Read the model definition and answer for the solid it produces. Units are mm, in the model's axes. Face numbers are marked on the shaded views. A direction names the side the tool comes from. Coordinates: 2 decimals unless noted, no trailing zeros. Write each loop counter-clockwise with the first axis right and the second up, starting at its lowest first coordinate (ties: lowest second). Pieces come first, ordered by that corner, then holes. Notation, with made-up numbers: M -9,-22 L 29,-22 A16 cw 29,-6 Z; hole C 23.25,31 d4. An arc over 180 degrees is marked long. Write item = value, one per line.
Autodesk Inventor part; units mm, degrees
ref_plane "YZ Plane" through (0, 0, 0) normal (1, 0, 0) x (0, 1, 0)
ref_plane "XZ Plane" through (0, 0, 0) normal (0, 1, 0) x (-1, 0, 0)
ref_plane "XY Plane" through (0, 0, 0) normal (0, 0, 1) x (1, 0, 0)
sketch "Skizze1" plane through (0, 0, 0) normal (0, 1, 0) x (-1, 0, 0)
  circle A0 centre (36.1244, -29.8236) radius 25
  circle A1 centre (36.1244, -29.8236) radius 1.5
  circle A2 centre (36.1244, -29.8236) radius 20
  point P0 (0, 0)
  dimension "d0" = 50
  dimension "d1" = 40
  dimension "d2" = 3
extrude "Extrusion1" add sketch "Skizze1" along normal blind 5 and the other way blind 5 contours A0
extrude "Extrusion2" add sketch "Skizze1" along normal blind 2.5 and the other way blind 2.5 contours A2
properties part number "Rad"
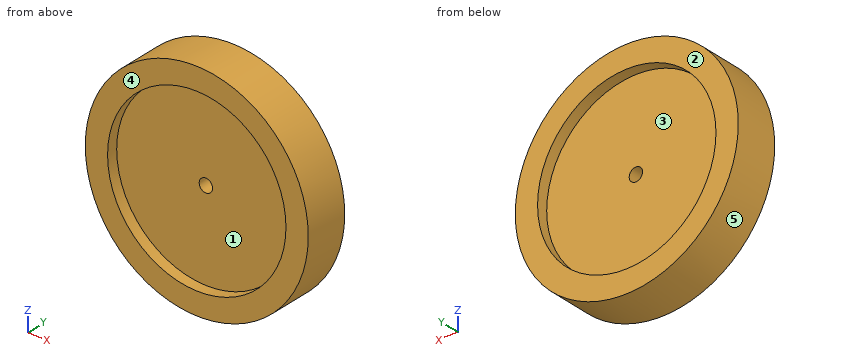
Item 1: Find section B-B (x = -30). Determine the outline of the cut face in (y, z).
Worked answers:
outline = M -5,-54.06 L 5,-54.06 L 5,-48.86 L 2.5,-48.86 L 2.5,-10.78 L 5,-10.78 L 5,-5.59 L -5,-5.59 L -5,-10.78 L -2.5,-10.78 L -2.5,-48.86 L -5,-48.86 Z
Item 2: Find section D-D (y = 1.5). Determine the outline of the cut face in (x, z), and give its area (3 significant figures).
Worked answers:
outline = C -36.12,-29.82 d50; hole C -36.12,-29.82 d3
area = 1,960 mm²
Item 3: Find section C-C (y = 4). Determine the outline of the cut face in (x, z).
Worked answers:
outline = C -36.12,-29.82 d50; hole C -36.12,-29.82 d40
Item 4: For a pull along Z with two mould halves and no side action, classify the marked faces 3, 4 and 5 as released by +Z, released by -Z, zero draft, split by the parting line, or undercut.
Worked answers:
face_3 = undercut
face_4 = zero draft
face_5 = split by the parting line
Item 5: Find section A-A (z = -35.5). Determine the outline of the cut face in (x, y).
Worked answers:
outline = M -60.47,-5 L -55.3,-5 L -55.3,-2.5 L -16.95,-2.5 L -16.95,-5 L -11.78,-5 L -11.78,5 L -16.95,5 L -16.95,2.5 L -55.3,2.5 L -55.3,5 L -60.47,5 Z
Item 6: Consider line 1 along Y through (x, z) = (-44, -31); line 2 along X through (y, z) = (-0.5, -29); line 3 along Z through (x, y) = (-47, -3.75). Determine where each line is inside the solid, lowest interval first. Write a range as from..to.
Worked answers:
line_1 = -2.5..2.5
line_2 = -61.11..-37.38, -34.87..-11.14
line_3 = -52.33..-46.61, -13.04..-7.31
Item 7: Which of the six approach directions +Z, -Z, +X, -X, +Y, -Y give full straight-line access (tool end or side, diameter ignored) to the marked faces 1 and 2?
Worked answers:
face_1 = -Y
face_2 = +Z, -Z, +X, -X, +Y
Item 8: Flat-ended cylindrical pins translate along their axes: pin 1 (2 mm diameter, centred on x = -29, z = -36, fed in from -Y); pin 2 (3 mm diameter, centred on x = -23, y = -3.5, fed in from +Z); pin 3 (1 mm diameter, centred on x = -40, y = 0, fed in from -Z); pin 4 (1.8 mm diameter, centred on x = -36.12, z = -29.82, fed in from -Y). Find the tip coordinate at first contact, or state that the pin passes through.
Worked answers:
pin_1 = -2.5
pin_2 = -7.69
pin_3 = -54.59
pin_4 = through
